from build123d import *

# Parameters (mm, degrees)
F0_R          = 6.9215
F0_R_2        = 3.2131
F1_DEPTH      = 5.588
F3_DEPTH      = 6.9225
F3_DEPTH_BACK = 6.9225
F4_R          = 2.54


with BuildPart() as f1:
    # F0 (on Top) → F1 (new body)
    with BuildSketch(Plane.XY):
        Circle(F0_R)
        Circle(F0_R_2, mode=Mode.SUBTRACT)
    extrude(amount=F1_DEPTH)

    # F2 (on Front) → F3 (cut, two sides)
    with BuildSketch(Plane.XZ) as f3_sk:
        with BuildLine():
            Line((4.7625, 5.588), (-4.7625, 5.588))
            ThreePointArc((-4.7625, 5.588), (0, 4.318), (4.7625, 5.588))
        make_face()
    extrude(amount=-F3_DEPTH, mode=Mode.SUBTRACT)
    extrude(f3_sk.sketch, amount=F3_DEPTH_BACK, mode=Mode.SUBTRACT)

    # F4
    f4_edges = [f1.edges().sort_by_distance(p)[0] for p in [
        (-4.7625, 0, 5.588),
        (4.7625, 0, 5.588),
    ]]
    fillet(f4_edges, radius=F4_R)


solid = f1.part
The listing builds one solid part. Answer for the finished solid, in the listing's coordinates (mm). A direction names the side the tool comes from. Coordinates: 2 decimals unless noted, no trailing zeros. Loops run counter-clockwise (first coordinate to the right, second up) from the corner with the lowest first, then second, coordinate; pieces in that order, holes last.
1) A tool of negligible diameter and unlimited length cuts with its end or side. For faces 4 (the face through (4.81, -0.08, 5.52)), 5 (the face through (-3.21, 0.14, 2.4)), from which of +Z, -Z, +X, -X, +Y, -Y can it reach the whole face along a straight path? Write none if from no direction.
2) Find section B-B on y = 0. Write down the section's boundary in (x, z), then the cut area to 3 significant figures.
3) Find section A-A on x = 0. Write down the section's boundary in (y, z).
4) A flat-ended cylindrical pin translates along its axis: pin 1 Ø1 at (y, z) = (3, 4.5) entering from +X. Find the tip coordinate at first contact, or state that the pin passes through.
5) Find section C-C on z = 3.55. Write down the section's boundary in (x, y), then the cut area to 3 significant figures.
6) Find the intervals of material crossed by L1, parallel to Y at x = 0, z = 3.55; L2, parallel to Y at x = -1.5, z = 3.5, in increasing order.
7) Determine the mould class of faces 1 (the face through (3, 2, 0)), 2 (the face through (-6.915, 0.304, 2.755)), 3 (the face through (-3, 1.6, 4.8)) for opening direction X: pulls with the +X half, pulls with the -X half, needs draft (parallel to the pull), parting line crosses it, or undercut.
8) Find section D-D on y = -3.5. Write down the section's boundary in (x, z), then the cut area to 3 significant figures.
Values:
1. face 4: +Z, +Y, -Y
1. face 5: +Z, -Z
2. outline: (-6.92, 0) - (-3.21, 0) - (-3.21, 4.87) arc R9.56 cw to (-4.26, 5.32) arc R2.54 ccw to (-5.4, 5.59) - (-6.92, 5.59) - close; (3.21, 0) - (6.92, 0) - (6.92, 5.59) - (5.4, 5.59) arc R2.54 ccw to (4.26, 5.32) arc R9.56 cw to (3.21, 4.87) - close
2. area: 40.2 mm2
3. outline: (-6.92, 0) - (-3.21, 0) - (-3.21, 4.32) - (-6.92, 4.32) - close; (3.21, 0) - (6.92, 0) - (6.92, 4.32) - (3.21, 4.32) - close
4. pin 1: stops at x = 6.45
5. outline: circle Ø13.84 at (0, 0); hole circle Ø6.43 at (0, 0)
5. area: 118 mm2
6. L1: y = -6.92 to -3.21, 3.21 to 6.92
6. L2: y = -6.76 to -2.84, 2.84 to 6.76
7. face 1: needs draft
7. face 2: parting line crosses it
7. face 3: undercut
8. outline: (-5.97, 0) - (5.97, 0) - (5.97, 5.59) - (5.4, 5.59) arc R2.54 ccw to (4.26, 5.32) arc R9.56 cw to (-4.26, 5.32) arc R2.54 ccw to (-5.4, 5.59) - (-5.97, 5.59) - close
8. area: 58.5 mm2
